from build123d import *

# Parameters (mm, degrees)
BOSS_EXTRUDE1_DEPTH = 25.4
SKETCH2_R           = 3.175
SKETCH2_R_2         = 0.79375
CUT_EXTRUDE1_DEPTH  = 25.4


with BuildPart() as part:
    # Sketch1 → Boss-Extrude1 (new body)
    with BuildSketch(Plane.XY):
        with BuildLine():
            Line((19.05, 50.8), (19.05, -50.8))
            ThreePointArc((19.05, -50.8), (0, -69.85), (-19.05, -50.8))
            Line((-19.05, -50.8), (-19.05, 50.8))
            ThreePointArc((-19.05, 50.8), (0, 69.85), (19.05, 50.8))
        make_face()
    extrude(amount=BOSS_EXTRUDE1_DEPTH)

    # Sketch2 → Cut-Extrude1 (cut)
    with BuildSketch(Plane.XY.offset(25.4)):
        with Locations((0, 50.8)):
            Circle(SKETCH2_R)
        with Locations((-4.939140867, 55.739140867)):
            Circle(SKETCH2_R_2)
        with Locations((-4.939140867, 45.860859133)):
            Circle(SKETCH2_R_2)
        with Locations((4.939140867, 55.739140867)):
            Circle(SKETCH2_R_2)
        with Locations((4.939140867, 45.860859133)):
            Circle(SKETCH2_R_2)
    cut_extrude1 = extrude(amount=-CUT_EXTRUDE1_DEPTH, mode=Mode.SUBTRACT)

    # Mirror1: Cut-Extrude1 across plane
    add(cut_extrude1.mirror(Plane.ZX), mode=Mode.SUBTRACT)


solid = part.part
For this review, take the finished solid that the model builds, in its own axes (mm). Round coordinates to 2 decimals unless told otherwise and drop trailing zeros. Write each loop counter-clockwise with the first axis right and the second up, starting at its lowest first coordinate (ties: lowest second). Pieces come first, ordered by that corner, then holes. Notation, with made-up numbers: (64.25, 15) - (115.25, 15) arc R30 cw to (115.25, 50) - close; hole circle Ø2 at (-23, 11). An arc over 180 degrees is marked (long way). Use a Markdown table: item, result.
Q1. The part is to be moulded in two halves that separate along X. For faces 1 (the flat face through (0, 1, 25.4)), 2 (the flat face through (-19.05, -1, 13)), 3 (the cylindrical face through (-0.41, 53.95, 12.88)), say which applies: pulls with the +X half, pulls with the -X half, needs draft (parallel to the pull), parting line crosses it, or undercut.
Derived:
| item | result |
|---|---|
| face 1 | needs draft |
| face 2 | pulls with the -X half |
| face 3 | undercut |
Q2. We need section C-C (y = 52). Give the boundary of the cut face in (x, z), plus the area to 3 significant figures.
Derived:
| item | result |
|---|---|
| outline | (-19.01, 0) - (-2.94, 0) - (-2.94, 25.4) - (-19.01, 25.4) - close; (2.94, 0) - (19.01, 0) - (19.01, 25.4) - (2.94, 25.4) - close |
| area | 816 mm2 |
Q3. We need section D-D (x = -9.5). Give the boundary of the cut face in (y, z).
Derived:
| item | result |
|---|---|
| outline | (-67.31, 0) - (67.31, 0) - (67.31, 25.4) - (-67.31, 25.4) - close |
Q4. Clearance check with flat-ended pins moving along their axes: pin 1 (1.4 mm diameter, centred on x = -4.94, y = 55.74, fed in from +Z); pin 2 (2 mm diameter, centred on x = -11.5, z = 14, fed in from -Y); pin 3 (10 mm diameter, centred on x = 11.5, z = 13.5, fed in from -Y). State where each tip first meets the part, or that it passes through.
Derived:
| item | result |
|---|---|
| pin 1 | passes through |
| pin 2 | stops at y = -66.7 |
| pin 3 | stops at y = -68.71 |
Q5. Wall thickness on line 1 along Y through (x, z) = (0, 8.75) (3 decimals); line 2 along Y through (x, z) = (4.5, 13.25); line 3 along X through (y, z) = (-50.8, 14.5) (3 decimals): over which ranges is each line inside the solid? List them lowest first.
Derived:
| item | result |
|---|---|
| line 1 | y = -69.85 to -53.975, -47.625 to 47.625, 53.975 to 69.85 |
| line 2 | y = -69.31 to -56.4, -55.08 to -46.52, -45.2 to 45.2, 46.52 to 55.08, 56.4 to 69.31 |
| line 3 | x = -19.05 to -3.175, 3.175 to 19.05 |
Q6. We need section B-B (z = 21.5). State how many separate pieces and enclosed holes the cut face has, plus the area to 3 significant figures.
Derived:
| item | result |
|---|---|
| separate pieces | 1 |
| enclosed holes | 10 |
| area | 4,930 mm2 |
Q7. We need section A-A (x = 0). Give the boundary of the cut face in (y, z) (3 decimals).
Derived:
| item | result |
|---|---|
| outline | (-69.85, 0) - (-53.975, 0) - (-53.975, 25.4) - (-69.85, 25.4) - close; (-47.625, 0) - (47.625, 0) - (47.625, 25.4) - (-47.625, 25.4) - close; (53.975, 0) - (69.85, 0) - (69.85, 25.4) - (53.975, 25.4) - close |
